Read the model definition and answer for the solid it produces. Units are mm, in the model's axes. Coordinates: 2 decimals unless noted, no trailing zeros. Order: outer loops, then holes, each group sorted by start corner. A loop starts at its lowest first (then second) coordinate and runs counter-clockwise, first axis right, second up. Notation, with made-up numbers: (43, 23) -> (78, 23) arc R22 ccw to (78, 33) -> close; hole circle Ø11 at (37.25, 11). An arc over 180 degrees is marked (long way). Answer as a JSON object with one key per item and string values. Group by question number.
1) Consider L1, parallel to Z at x = -42.5, y = 58.5; L2, parallel to Y at x = -51, z = 34; L3, parallel to Y at x = -48.5, z = 69.5 (3 decimals). Determine where each line is inside the solid, lowest interval first.
2) Section A-A on z = 102.5 is taken. Determine the outline of the cut face in (x, y).
3) Section B-B on y = 74.5 is taken. Determine the outline of the cut face in (x, z).
4) Section C-C on x = -35.5 is taken. Determine the outline of the cut face in (y, z).
5) Given pin 1 (8 mm diameter, centred on y = 64, z = 25, fed in from +X); pin 2 (1 mm diameter, centred on y = 69.5, z = 66.5, fed in from +X); pin 3 (5 mm diameter, centred on x = -58.5, y = 85, fed in from -Z), each flat-ended and moving along its own axis, determine where each tip first touches the part or whether it passes through.
from build123d import *

# Parameters (mm, degrees)
SKETCH_1_R          = 1.75
EXTRUDE_1_DEPTH     = 135.293792798
SKETCH_3_W          = 133.999999999
SKETCH_3_H          = 92.793140679
CUT_EXTRUDE_1_DEPTH = 210.099404157


with BuildPart() as part:
    # 草图1 → 凸台-拉伸1 (new body)
    with BuildSketch(Plane.XY):
        with BuildLine():
            Line((-17.129972102, 49.08105856), (-8.373318144, 72.720547785))
            Line((-8.373318144, 72.720547785), (-46.360961782, 136.227129066))
            ThreePointArc((-46.360961782, 136.227129066), (-48.203989789, 137.596554385), (-50.47553732, 137.261666712))
            Line((-50.47553732, 137.261666712), (-77.638405872, 121.013691307))
            ThreePointArc((-77.638405872, 121.013691307), (-79.007831191, 119.1706633), (-78.672943518, 116.899115769))
            Line((-78.672943518, 116.899115769), (-40.908434768, 53.765564573))
            ThreePointArc((-40.908434768, 53.765564573), (-40.714211977, 53.380474511), (-40.57721581, 52.971513757))
            Line((-40.57721581, 52.971513757), (-38.440433205, 44.648087586))
            Line((-38.440433205, 44.648087586), (-17.486445488, 57.181732929))
            Line((-17.486445488, 57.181732929), (-18.690847722, 47.397023253))
            ThreePointArc((-18.690847722, 47.397023253), (-17.742918238, 48.083798514), (-17.129972102, 49.08105856))
        make_face()
        with Locations(Location((-71.983811388, 117.404597068, 0), (0, 0, 90))):
            Circle(SKETCH_1_R, mode=Mode.SUBTRACT)
        with Locations(Location((-49.970056021, 130.572534582, 0), (0, 0, 90))):
            Circle(SKETCH_1_R, mode=Mode.SUBTRACT)
    extrude(amount=EXTRUDE_1_DEPTH)

    # 草图3 → 切除-拉伸1 (cut, through all)
    with BuildSketch(Plane(origin=(14.886439913, 8.904336531, 0), x_dir=(0, 0, -1), z_dir=(0.8581922502722595, 0.5133284149281387, 0))):
        with Locations((-65.293792798, 97.310855858)):
            Rectangle(SKETCH_3_W, SKETCH_3_H)
    extrude(amount=-CUT_EXTRUDE_1_DEPTH, mode=Mode.SUBTRACT)


solid = part.part
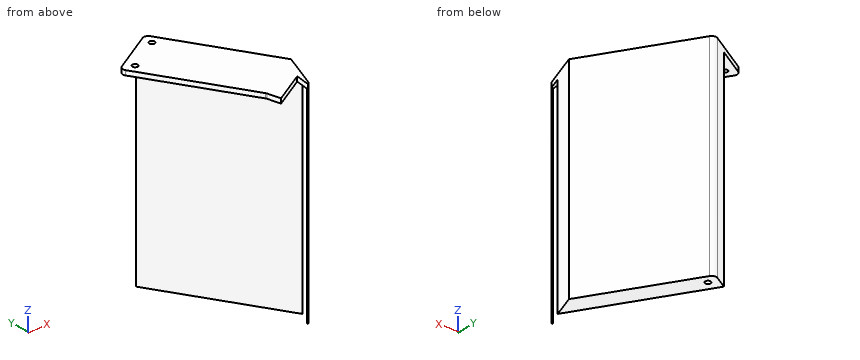
Worked answers:
{
 "1": {"L1": "z = 132.29 to 135.29", "L2": "y = 119.05 to 129.16, 131.99 to 136.95", "L3": "y = 114.875 to 129.623, 131.522 to 137.655"},
 "2": {"outline": "(-58.88, 132.23) -> (-14.08, 57.32) -> (-8.37, 72.72) -> (-46.36, 136.23) arc R3 ccw to (-50.48, 137.26) -> close; (-18.69, 47.4) arc R3 ccw to (-17.13, 49.08) -> (-18.59, 48.21) -> close; hole circle Ø3.5 at (-49.97, 130.57)"},
 "3": {"outline": "(-53.31, 132.29) -> (-24.35, 132.29) -> (-24.35, 0) -> (-9.44, 0) -> (-9.44, 135.29) -> (-53.31, 135.29) -> close"},
 "4": {"outline": "(46.41, 132.29) -> (93.14, 132.29) -> (93.14, 0) -> (118.07, 0) -> (118.07, 135.29) -> (46.41, 135.29) -> close"},
 "5": {"pin 1": "stops at x = -10.12", "pin 2": "stops at x = -9.38", "pin 3": "stops at z = 132.29"}
}
